from build123d import *

# Parameters (mm, degrees)
SKETCH1_R                   = 16
BOSS_EXTRUDE1_DEPTH         = 38
SKETCH2_R                   = 13.8
BOSS_EXTRUDE2_DEPTH         = 38
SKETCH3_R                   = 5
BOSS_EXTRUDE3_DEPTH         = 2
SKETCH4_R                   = 10
BOSS_EXTRUDE4_DEPTH         = 3
SKETCH5_R                   = 3
BOSS_EXTRUDE5_DEPTH         = 16
TAP_DRILL_FOR_M3_TAP1_D     = 2.5
TAP_DRILL_FOR_M3_TAP1_DEPTH = 5
TAP_DRILL_FOR_M3_TAP1_TIP   = 0.751075774
TAP_DRILL_FOR_M3_TAP2_D     = 2.5
TAP_DRILL_FOR_M3_TAP2_DEPTH = 5
TAP_DRILL_FOR_M3_TAP2_TIP   = 0.751075774


with BuildPart() as part:
    # Sketch1 → Boss-Extrude1 (new body)
    with BuildSketch(Plane.XY):
        Circle(SKETCH1_R)
    extrude(amount=BOSS_EXTRUDE1_DEPTH)

    # Sketch2 → Boss-Extrude2 (add)
    with BuildSketch(Plane(origin=(0, 0, 0), x_dir=(-1, 0, 0), z_dir=(0, 0, -1))):
        Circle(SKETCH2_R)
    extrude(amount=BOSS_EXTRUDE2_DEPTH)

    # Sketch3 → Boss-Extrude3 (add)
    with BuildSketch(Plane(origin=(0, 0, -38), x_dir=(-1, 0, 0), z_dir=(0, 0, -1))):
        Circle(SKETCH3_R)
    extrude(amount=BOSS_EXTRUDE3_DEPTH)

    # Sketch4 → Boss-Extrude4 (add)
    with BuildSketch(Plane.XY.offset(38)):
        Circle(SKETCH4_R)
    extrude(amount=BOSS_EXTRUDE4_DEPTH)

    # Sketch5 → Boss-Extrude5 (add)
    with BuildSketch(Plane.XY.offset(41)):
        Circle(SKETCH5_R)
    extrude(amount=BOSS_EXTRUDE5_DEPTH)

    # Tap Drill for M3 Tap1
    with Locations(Plane(origin=(0, 0, -38), x_dir=(-1, 0, 0), z_dir=(0, 0, -1))):
        with Locations((-13, 0), (0, -13), (13, 0), (0, 13)):
            Hole(TAP_DRILL_FOR_M3_TAP1_D / 2, depth=TAP_DRILL_FOR_M3_TAP1_DEPTH)
            with Locations((0, 0, -(TAP_DRILL_FOR_M3_TAP1_DEPTH + TAP_DRILL_FOR_M3_TAP1_TIP / 2))):  # 118° drill point
                Cone(0, TAP_DRILL_FOR_M3_TAP1_D / 2, TAP_DRILL_FOR_M3_TAP1_TIP, mode=Mode.SUBTRACT)

    # Tap Drill for M3 Tap2
    with Locations(Plane.XY.offset(38)):
        with Locations((0, 13), (-13, 0), (0, -13), (13, 0)):
            Hole(TAP_DRILL_FOR_M3_TAP2_D / 2, depth=TAP_DRILL_FOR_M3_TAP2_DEPTH)
            with Locations((0, 0, -(TAP_DRILL_FOR_M3_TAP2_DEPTH + TAP_DRILL_FOR_M3_TAP2_TIP / 2))):  # 118° drill point
                Cone(0, TAP_DRILL_FOR_M3_TAP2_D / 2, TAP_DRILL_FOR_M3_TAP2_TIP, mode=Mode.SUBTRACT)


solid = part.part
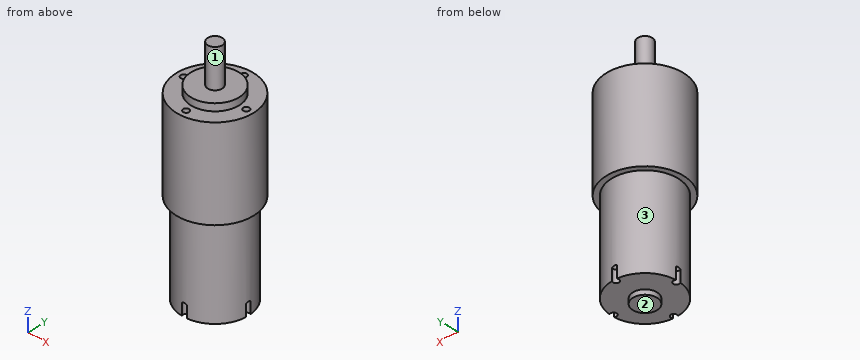
Verification items for the finished model (mm, model axes). Face numbers are marked on the shaded views. A direction names the side the tool comes from. Round coordinates to 2 decimals unless told otherwise and drop trailing zeros. Loops run counter-clockwise (first coordinate to the right, second up) from the corner with the lowest first, then second, coordinate; pieces in that order, holes last. Notation, with made-up numbers: (40.5, 52.5) - (81.5, 52.5) arc R20 cw to (81.5, 75.5) - close; hole circle Ø6 at (38.25, 52.5). An arc over 180 degrees is marked (long way). Use a Markdown table: item, result. Add a question column.
1. Section check A-A, the plane y = 8.5. Record the boundary of the cut face in (x, z).
2. Section check C-C, the plane z = 6. Record the boundary of the cut face in (x, y).
3. Access from +Z, -Z, +X, -X, +Y, -Y to the whole of each face (thin tool, end or side, straight path). Record for the marked faces 1, 2 and 3.
4. Gauge pin test, flat ends, axial feed: pin 1 (2 mm diameter, centred on x = -13, y = 0, fed in from -Z); pin 2 (2 mm diameter, centred on x = -13, y = 0, fed in from +Z); pin 3 (3 mm diameter, centred on x = 0, y = -13, fed in from -Z). Record the tip position at first contact, or that the pin passes through.
5. Section check B-B, the plane x = -9. Record the boundary of the cut face in (y, z).
6. Thickness scan on probe 1 along Y at (x, z) = (0, 35); probe 2 along Z at (x, y) = (7, 3.5); probe 3 along Y at (x, z) = (-13, 36). Record the ranges inside material, lowest first. Write a range as [from, to].
Checks:
| question | item | result |
|---|---|---|
| 1 | outline | (-13.56, 0) - (-10.87, 0) - (-10.87, -38) - (10.87, -38) - (10.87, 0) - (13.56, 0) - (13.56, 38) - (5.27, 38) - (5.27, 41) - (-5.27, 41) - (-5.27, 38) - (-13.56, 38) - close |
| 2 | outline | circle Ø32 at (0, 0) |
| 3 | face 1 | +Z |
| 3 | face 2 | -Z, +X, -X, +Y, -Y |
| 3 | face 3 | -Z |
| 4 | pin 1 | stops at z = -32.85 |
| 4 | pin 2 | stops at z = 32.85 |
| 4 | pin 3 | stops at z = -38 |
| 5 | outline | (-13.23, 0) - (-10.46, 0) - (-10.46, -38) - (10.46, -38) - (10.46, 0) - (13.23, 0) - (13.23, 38) - (4.36, 38) - (4.36, 41) - (-4.36, 41) - (-4.36, 38) - (-13.23, 38) - close |
| 6 | probe 1 | y = [-16, -14.25], [-11.75, 11.75], [14.25, 16] |
| 6 | probe 2 | z = [-38, 41] |
| 6 | probe 3 | y = [-9.33, -1.25], [1.25, 9.33] |
